from build123d import *


with BuildPart() as part:
    # 草图1 → 旋转1 (revolve)
    with BuildSketch(Plane.XY, mode=Mode.PRIVATE) as revolve_1_sk:
        Polygon((19.05, 0), (19.05, 12.7), (17, 12.7), (17, 13.7), (17.5, 13.7), (17.5, 17.7), (15, 17.7), (15, 5.5), (17.6, 5.5), (17.6, 4.5), (17, 4.5), (17, 0), align=None)
    revolve(revolve_1_sk.sketch.rotate(Axis((0, 161.376166943, 0), (0, -1, 0)), 90), axis=Axis((0, 161.376166943, 0), (0, -1, 0)))  # turned: the seam where the file's is


solid = part.part
Here's how the part is built. I have some questions about the finished solid (model axes, mm). A direction names the side the tool comes from. Give positions to 0.01 mm unless a question says otherwise; leave off trailing zeros. Order: outer loops, then holes, each group sorted by start corner. A loop starts at its lowest first (then second) coordinate and runs counter-clockwise, first axis right, second up. Notation, with made-up numbers: (-12, 64.5) -> (16, 64.5) arc R21 cw to (16, 78.5) -> close; hole circle Ø3 at (-32, -18). An arc over 180 degrees is marked (long way). Use a Markdown table: item, result. Add a question column.
Item 1: Imagine slicing it at D-D on x = 16.5. Please give me the cut outline in (y, z).
Item 2: Imagine slicing it at B-B on z = 0. Please give me the cut outline in (x, y).
Item 3: For faces 1 (the face through (-17.45, 4.99, -2.29)), 2 (the face through (-16.855, 2.218, -2.213)), 3 (the face through (-16, 0, 7)), which set-ups out of +Z, -Z, +X, -X, +Y, -Y let a thin tool reach every point of the face, with its end or its side?
Item 4: If we mould it in two halves opening along Z, with no side actions, what happens to faces 4 (the face through (-12.65, 11.51, 8.06)), 5 (the face through (17.084, 15.728, -3.794)), 6 (the face through (-16, 12.7, -7)), 7 (the face through (-8, 5.5, -13))? For each: pulls with the +Z half, pulls with the -Z half, needs draft (parallel to the pull), parting line crosses it, or undercut.
Item 5: Imagine slicing it at C-C on y = 3.25. Please give me the cut outline in (x, z), plus the area to 3 significant figures.
Item 6: Imagine slicing it at A-A on x = 0. Please give me the cut outline in (y, z), plus the area to 3 significant figures.
Item 7: I need wall thicknesses on line 1 (X direction, y = 1.85, z = 0); line 2 (X direction, y = 4.8, z = 0); line 3 (Z direction, x = 11, y = 14.25). Which ranges of each line are inside material? Lowest first, please.
Item 8: Will these pins go through, and if not, where does the flat tip stop? pin 1 (21 mm diameter, centred on x = 0, z = 0, fed in from -Y); pin 2 (17.5 mm diameter, centred on x = -1, z = 6.5, fed in from -Y); pin 3 (3 mm diameter, centred on x = 1, y = 15.5, fed in from -Z); pin 4 (3 mm diameter, centred on x = 9, y = 13, fed in from +Z).
Data:
| question | item | result |
|---|---|---|
| 1 | outline | (0, -9.52) -> (12.7, -9.52) -> (12.7, -4.09) -> (13.7, -4.09) -> (13.7, -5.83) -> (17.7, -5.83) -> (17.7, 5.83) -> (13.7, 5.83) -> (13.7, 4.09) -> (12.7, 4.09) -> (12.7, 9.52) -> (0, 9.52) -> (0, 4.09) -> (4.5, 4.09) -> (4.5, 6.12) -> (5.5, 6.12) -> (5.5, -6.12) -> (4.5, -6.12) -> (4.5, -4.09) -> (0, -4.09) -> close |
| 2 | outline | (-19.05, 0) -> (-17, 0) -> (-17, 4.5) -> (-17.6, 4.5) -> (-17.6, 5.5) -> (-15, 5.5) -> (-15, 17.7) -> (-17.5, 17.7) -> (-17.5, 13.7) -> (-17, 13.7) -> (-17, 12.7) -> (-19.05, 12.7) -> close; (15, 5.5) -> (17.6, 5.5) -> (17.6, 4.5) -> (17, 4.5) -> (17, 0) -> (19.05, 0) -> (19.05, 12.7) -> (17, 12.7) -> (17, 13.7) -> (17.5, 13.7) -> (17.5, 17.7) -> (15, 17.7) -> close |
| 3 | face 1 | none |
| 3 | face 2 | -Y |
| 3 | face 3 | +Z, -Z, +X, -X, -Y |
| 4 | face 4 | undercut |
| 4 | face 5 | parting line crosses it |
| 4 | face 6 | needs draft |
| 4 | face 7 | undercut |
| 5 | outline | circle Ø38.1 at (0, 0); hole circle Ø34 at (0, 0) |
| 5 | area | 232 mm² |
| 6 | outline | (0, -19.05) -> (12.7, -19.05) -> (12.7, -17) -> (13.7, -17) -> (13.7, -17.5) -> (17.7, -17.5) -> (17.7, -15) -> (5.5, -15) -> (5.5, -17.6) -> (4.5, -17.6) -> (4.5, -17) -> (0, -17) -> close; (0, 17) -> (4.5, 17) -> (4.5, 17.6) -> (5.5, 17.6) -> (5.5, 15) -> (17.7, 15) -> (17.7, 17.5) -> (13.7, 17.5) -> (13.7, 17) -> (12.7, 17) -> (12.7, 19.05) -> (0, 19.05) -> close |
| 6 | area | 104 mm² |
| 7 | line 1 | x = -19.05 to -17, 17 to 19.05 |
| 7 | line 2 | x = -19.05 to -17.6, 17.6 to 19.05 |
| 7 | line 3 | z = -13.61 to -10.2, 10.2 to 13.61 |
| 8 | pin 1 | passes through |
| 8 | pin 2 | stops at y = 5.5 |
| 8 | pin 3 | stops at z = -17.5 |
| 8 | pin 4 | stops at z = 17.5 |
